Build history of the part. All positions in model axes, mm. Give positions to 0.01 mm unless a question says otherwise; leave off trailing zeros. Order: outer loops, then holes, each group sorted by start corner. A loop starts at its lowest first (then second) coordinate and runs counter-clockwise, first axis right, second up. Notation, with made-up numbers: (20, 36.25) -> (24, 36.25) arc R12 ccw to (24, 58.25) -> close; hole circle Ø1 at (-6.5, -32). An arc over 180 degrees is marked (long way). One line per question, with ' | ' between items. Start each with the question number.
(1) Pin check, flat tips, straight feed: pin 1 Ø1.5 at (y, z) = (4, -10) entering from -X; pin 2 Ø4 at (x, y) = (-18.5, 2.5) entering from +Z; pin 3 Ø6 at (y, z) = (5, -3.5) entering from -X (3 decimals). Stop position of each tip, or through.
(2) Cut at B-B (z = 0). Give the cut face in (x, y).
(3) Cut at A-A (y = 8). Give the number of separate pieces and of enclosed holes in the cut face, then the cut area to 3 significant figures.
(4) Cut at D-D (x = 0). Give the cut face in (y, z), then the cut area to 3 significant figures.
(5) Pull direction X, two halves, no side cores. Call faces 1 (the face through (7.509, 4.93, 23.846)), 2 (the face through (-5, 0, 0)), 3 (the face through (0.191, 4.93, -14.353)): +X half, -X half, draft (parallel to the pull), parting line (faces both ways), or undercut.
(6) Drill centre lines: L1, parallel to X at y = 4.25, z = 17.5; L2, parallel to Z at x = 4, y = 4.5; L3, parallel to Z at x = 0, y = 7.5. Where is each one in solid material? Low to high. Write a range as from..to.
(7) Cut at C-C (x = 16). Give the cut face in (y, z).
from build123d import *

# Parameters (mm, degrees)
BASE_REFERENCE_SKETCH_R       = 25
BASE_REFERENCE_SKETCH_R_2     = 1.5
BASE_WHEEL_EXTRUDE_DEPTH      = 10
SPOKES_CIRCULAR_PATTERN_COUNT = 7
M2_CLEARANCE_HOLE1_D          = 2.4
CIRPATTERN1_COUNT             = 2


with BuildPart() as part:
    # Base Reference Sketch → Base Wheel Extrude (new body)
    with BuildSketch(Plane(origin=(0, 0, 0), x_dir=(1, 0, 0), z_dir=(0, 1, 0))):
        with Locations(Location((0, 0, 0), (0, 0, 270))):
            Circle(BASE_REFERENCE_SKETCH_R)
        with BuildLine():
            ThreePointArc((-6.099694515, 19.047144847), (11.877442501, -16.091188882), (-16.404494382, 11.440828819))
            ThreePointArc((-16.404494382, 11.440828819), (-7.848653173, 14.358553237), (-2.5, 7.071067812))
            ThreePointArc((-2.5, 7.071067812), (0, -7.5), (2.5, 7.071067812))
            ThreePointArc((2.5, 7.071067812), (0.127377259, 14.442993729), (-6.099694515, 19.047144847))
        make_face(mode=Mode.SUBTRACT)
        with Locations(Location((0, 0, 0), (0, 0, 270))):
            Circle(BASE_REFERENCE_SKETCH_R_2, mode=Mode.SUBTRACT)
    base_wheel_extrude = extrude(amount=BASE_WHEEL_EXTRUDE_DEPTH)

    # Spokes Circular Pattern: Base Wheel Extrude ×7 about axis
    spokes_circular_pattern_axis = Axis((0, 0, 0), (0, 1, 0))
    for i in range(1, SPOKES_CIRCULAR_PATTERN_COUNT):
        add(base_wheel_extrude.rotate(spokes_circular_pattern_axis, i * 360 / SPOKES_CIRCULAR_PATTERN_COUNT))

    # M2 Clearance Hole1 (through all)
    with Locations(Plane(origin=(0, 0, 0), x_dir=(-1, 0, 0), z_dir=(0, -1, 0))):
        with Locations((0, 4)):
            m2_clearance_hole1 = Hole(M2_CLEARANCE_HOLE1_D / 2)

    # CirPattern1: M2 Clearance Hole1 ×2 about axis
    cirpattern1_axis = Axis((0, 0, 0), (0, 1, 0))
    for i in range(1, CIRPATTERN1_COUNT):
        add(m2_clearance_hole1.rotate(cirpattern1_axis, i * 360 / CIRPATTERN1_COUNT), mode=Mode.SUBTRACT)


solid = part.part
Result set:
1) pin 1: stops at x = -23.23 | pin 2: stops at z = 18.78 | pin 3: stops at x = -24.995
2) outline: (-25, 0) -> (-18.63, 0) -> (-18.63, 10) -> (-25, 10) -> close; (-9.97, 0) -> (-1.5, 0) -> (-1.5, 10) -> (-9.97, 10) -> close; (1.5, 0) -> (18.67, 0) -> (18.67, 10) -> (1.5, 10) -> close; (20, 0) -> (25, 0) -> (25, 10) -> (20, 10) -> close
3) separate pieces: 1 | enclosed holes: 10 | area: 1,420 mm2
4) outline: (0, -25) -> (10, -25) -> (10, -19.93) -> (0, -19.93) -> close; (0, -14.62) -> (10, -14.62) -> (10, -5.2) -> (0, -5.2) -> close; (0, -2.8) -> (10, -2.8) -> (10, -1.5) -> (0, -1.5) -> close; (0, 1.5) -> (10, 1.5) -> (10, 2.8) -> (0, 2.8) -> close; (0, 5.2) -> (10, 5.2) -> (10, 7.5) -> (0, 7.5) -> close; (0, 15.41) -> (10, 15.41) -> (10, 25) -> (0, 25) -> close | area: 290 mm2
5) face 1: parting line | face 2: draft | face 3: undercut
6) L1: x = -17.85..-9.31, -4.63..2.45, 9.68..17.85 | L2: z = -24.68..-18.28, -6.39..11.59, 18.12..24.68 | L3: z = -25..-19.93, -14.62..-5.2, -2.8..-1.5, 1.5..2.8, 5.2..7.5, 15.41..25
7) outline: (0, -19.21) -> (10, -19.21) -> (10, -11.69) -> (0, -11.69) -> close; (0, -4.93) -> (10, -4.93) -> (10, 2.31) -> (0, 2.31) -> close; (0, 8.6) -> (10, 8.6) -> (10, 19.21) -> (0, 19.21) -> close
